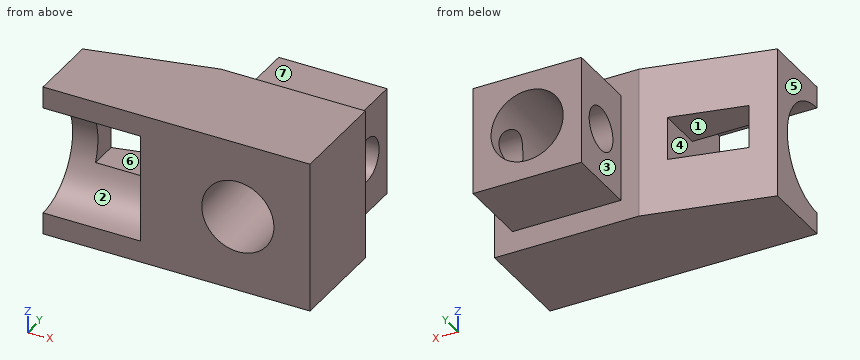
```python
from build123d import *

# Parameters (mm, degrees)
BOSS_EXTRUDE1_DEPTH = 42
SKETCH3_W           = 20
SKETCH3_H           = 12
CUT_EXTRUDE1_DEPTH  = 42
CUT_EXTRUDE2_DEPTH  = 45
SKETCH5_W           = 30
SKETCH5_H           = 20
CUT_EXTRUDE3_DEPTH  = 6
SKETCH6_W           = 30
SKETCH6_H           = 20
CUT_EXTRUDE4_DEPTH  = 6
CUT_EXTRUDE5_DEPTH  = 27
SKETCH8_R           = 6
CUT_EXTRUDE6_DEPTH  = 42
SKETCH9_R           = 7.5
CUT_EXTRUDE7_DEPTH  = 70
CUT_EXTRUDE8_DEPTH  = 27
SKETCH11_R          = 10
CUT_EXTRUDE9_DEPTH  = 58


with BuildPart() as part:
    # Sketch2 → Boss-Extrude1 (new body)
    with BuildSketch(Plane.XY):
        Polygon((0, 28), (39, 28), (39, 48), (69, 48), (69, 28), (74, 28), (74, 0), (0, 0), align=None)
    extrude(amount=BOSS_EXTRUDE1_DEPTH)

    # Sketch3 → Cut-Extrude1 (cut)
    with BuildSketch(Plane(origin=(0, 28, 0), x_dir=(1, 0, 0), z_dir=(0, 1, 0))):
        with Locations((17, -21)):
            Rectangle(SKETCH3_W, SKETCH3_H)
    extrude(amount=-CUT_EXTRUDE1_DEPTH, mode=Mode.SUBTRACT)

    # Sketch4 → Cut-Extrude2 (cut)
    with BuildSketch(Plane.XY.offset(42)):
        Polygon((0, 20), (34, 28), (0, 28), align=None)
    extrude(amount=-CUT_EXTRUDE2_DEPTH, mode=Mode.SUBTRACT)

    # Sketch5 → Cut-Extrude3 (cut)
    with BuildSketch(Plane.XY.offset(42)):
        with Locations((54, 38)):
            Rectangle(SKETCH5_W, SKETCH5_H)
    extrude(amount=-CUT_EXTRUDE3_DEPTH, mode=Mode.SUBTRACT)

    # Sketch6 → Cut-Extrude4 (cut)
    with BuildSketch(Plane(origin=(0, 0, 0), x_dir=(-1, 0, 0), z_dir=(0, 0, -1))):
        with Locations((-54, 38)):
            Rectangle(SKETCH6_W, SKETCH6_H)
    extrude(amount=-CUT_EXTRUDE4_DEPTH, mode=Mode.SUBTRACT)

    # Sketch7 → Cut-Extrude5 (cut)
    with BuildSketch(Plane.ZY):
        with BuildLine():
            ThreePointArc((13.5, 0), (21, -7.5), (28.5, 0))
            Line((28.5, 0), (13.5, 0))
        make_face()
        with BuildLine():
            Line((13.5, 0), (28.5, 0))
            ThreePointArc((28.5, 0), (21, 7.5), (13.5, 0))
        make_face()
    extrude(amount=-CUT_EXTRUDE5_DEPTH, mode=Mode.SUBTRACT)

    # Sketch8 → Cut-Extrude6 (cut)
    with BuildSketch(Plane.ZY.offset(-39)):
        with Locations((21, 38)):
            Circle(SKETCH8_R)
    extrude(amount=-CUT_EXTRUDE6_DEPTH, mode=Mode.SUBTRACT)

    # Sketch9 → Cut-Extrude7 (cut)
    with BuildSketch(Plane(origin=(0, 48, 0), x_dir=(1, 0, 0), z_dir=(0, 1, 0))):
        with Locations(Location((54, -21, 0), (0, 0, 270))):
            Circle(SKETCH9_R)
    extrude(amount=-CUT_EXTRUDE7_DEPTH, mode=Mode.SUBTRACT)

    # Sketch10 → Cut-Extrude8 (cut)
    with BuildSketch(Plane.ZY):
        with BuildLine():
            ThreePointArc((36, 0), (21, 15), (6, 0))
            Line((6, 0), (13.5, 0))
            ThreePointArc((13.5, 0), (21, 7.5), (28.5, 0))
            Line((28.5, 0), (36, 0))
        make_face()
        with BuildLine():
            Line((13.5, 0), (6, 0))
            ThreePointArc((6, 0), (21, -15), (36, 0))
            Line((36, 0), (28.5, 0))
            ThreePointArc((28.5, 0), (21, 7.5), (13.5, 0))
        make_face()
    extrude(amount=-CUT_EXTRUDE8_DEPTH, mode=Mode.SUBTRACT)

    # Sketch11 → Cut-Extrude9 (cut)
    with BuildSketch(Plane(origin=(0, 48, 0), x_dir=(1, 0, 0), z_dir=(0, 1, 0))):
        with Locations(Location((54, -21, 0), (0, 0, 270))):
            Circle(SKETCH11_R)
    extrude(amount=-CUT_EXTRUDE9_DEPTH, mode=Mode.SUBTRACT)


solid = part.part
```
Can you work these out from the model? Positions are in its coordinate system, mm. Face numbers are marked on the shaded views. A direction names the side the tool comes from. Coordinates: 2 decimals unless noted, no trailing zeros. Loops run counter-clockwise (first coordinate to the right, second up) from the corner with the lowest first, then second, coordinate; pieces in that order, holes last. Notation, with made-up numbers: (-30, 29) -> (-20, 29) arc R7 cw to (-20, 34) -> close; hole circle Ø9 at (-8.5, -38.5). An arc over 180 degrees is marked (long way). Answer as a JSON object with one key per item and string values.
1) Imagine slicing it at D-D (y = 38). Please give me the cut outline in (x, z), then the cut area to 3 significant figures.
Results:
{"outline": "(39, 6) -> (69, 6) -> (69, 15) -> (62, 15) arc R10 cw to (46, 15) -> (39, 15) -> close; (39, 27) -> (46, 27) arc R10 cw to (62, 27) -> (69, 27) -> (69, 36) -> (39, 36) -> close", "area": "451 mm^2"}
2) Imagine slicing it at C-C (x = 54). Please give me the cut outline in (y, z).
Results:
{"outline": "(0, 0) -> (28, 0) -> (28, 6) -> (48, 6) -> (48, 11) -> (0, 11) -> close; (0, 31) -> (48, 31) -> (48, 36) -> (28, 36) -> (28, 42) -> (0, 42) -> close"}
3) Thinking about a two-plate mould opening in X: for the marked faces 5, 6 and 7, which applies, pulls with the +X half, pulls with the -X half, needs draft (parallel to the pull), parting line crosses it, or undercut?
Results:
{"face 5": "pulls with the -X half", "face 6": "undercut", "face 7": "needs draft"}
4) For P1, Ø3, axis at x = 35, z = 18, coming from the +Y side; P2, Ø16, axis at x = 57.5, y = 33.5, coming from the -Z side; P3, Ø14, axis at y = 38, z = 21, coming from the +X side; P4, Ø16, axis at x = 49, y = 42.5, coming from the +Z side, each with a flat end and sliding along its axis, tell me the tip position at first contact or that it passes through.
Results:
{"P1": "stops at y = 28", "P2": "stops at z = 0", "P3": "stops at x = 69", "P4": "stops at z = 36"}
5) For the marked faces 1, 2, 3 and 4, which set-ups out of +Z, -Z, +X, -X, +Y, -Y let a thin tool reach every point of the face, with its end or its side?
Results:
{"face 1": "+Y, -Y", "face 2": "-X, -Y", "face 3": "+Z, -Z, -X, +Y", "face 4": "-Y"}
6) Imagine slicing it at A-A (z = 21). Please give me the cut outline in (x, y).
Results:
{"outline": "(0, 15) -> (7, 15) -> (7, 21.65) -> (0, 20) -> close; (27, 0) -> (44, 0) -> (44, 32) -> (39, 32) -> (39, 28) -> (34, 28) -> (27, 26.35) -> close; (39, 44) -> (44, 44) -> (44, 48) -> (39, 48) -> close; (64, 0) -> (74, 0) -> (74, 28) -> (69, 28) -> (69, 32) -> (64, 32) -> close; (64, 44) -> (69, 44) -> (69, 48) -> (64, 48) -> close"}
7) Imagine slicing it at B-B (y = 23). Please give me the cut outline in (x, z), then the cut area to 3 significant figures.
Results:
{"outline": "(12.75, 0) -> (74, 0) -> (74, 42) -> (12.75, 42) -> (12.75, 27) -> (27, 27) -> (27, 15) -> (12.75, 15) -> close; hole circle Ø20 at (54, 21)", "area": "2,090 mm^2"}
8) If I drill on line 1 (Y direction, x = 42.25, z = 21); line 2 (X direction, y = 12, z = 21); line 3 (Z direction, x = 42.75, y = 38), over which ranges is the centre line in solid material (lowest first)?
Results:
{"line 1": "y = 0 to 32, 44 to 48", "line 2": "x = 27 to 44, 64 to 74", "line 3": "z = 6 to 15, 27 to 36"}
